The model under review builds one solid part; all positions refer to its coordinate system, in mm. A direction names the side the tool comes from. Coordinates: 2 decimals unless noted, no trailing zeros. Order: outer loops, then holes, each group sorted by start corner. A loop starts at its lowest first (then second) coordinate and runs counter-clockwise, first axis right, second up.
from build123d import *

# Parameters (mm, degrees)
SKETCH_1_W      = 86
SKETCH_1_H      = 57.4
EXTRUDE_1_DEPTH = 1.6
SKETCH_2_W      = 84.66
SKETCH_2_H      = 54.44
EXTRUDE_2_DEPTH = 1.3
SKETCH_3_W      = 75.45
SKETCH_3_H      = 50.61
EXTRUDE_3_DEPTH = 0.1
SKETCH_4_W      = 51.17
SKETCH_4_H      = 5
EXTRUDE_4_DEPTH = 14


with BuildPart() as part:
    # 草图1 → 凸台-拉伸1 (new body)
    with BuildSketch(Plane(origin=(0, 0, 0), x_dir=(1, 0, 0), z_dir=(0, 1, 0))):
        with Locations((-1.791666667, -4.811111111)):
            Rectangle(SKETCH_1_W, SKETCH_1_H)
    extrude(amount=EXTRUDE_1_DEPTH)

    # 草图2 → 凸台-拉伸2 (add)
    with BuildSketch(Plane(origin=(0, 1.6, 0), x_dir=(1, 0, 0), z_dir=(0, 1, 0))):
        with Locations((-1.461666667, -4.611111111)):
            Rectangle(SKETCH_2_W, SKETCH_2_H)
    extrude(amount=EXTRUDE_2_DEPTH)

    # 草图3 → 凸台-拉伸3 (add)
    with BuildSketch(Plane(origin=(0, 2.9, 0), x_dir=(1, 0, 0), z_dir=(0, 1, 0))):
        with Locations((1.323333333, -4.516111111)):
            Rectangle(SKETCH_3_W, SKETCH_3_H)
    extrude(amount=EXTRUDE_3_DEPTH)

    # 草图4 → 凸台-拉伸4 (add)
    with BuildSketch(Plane.XZ):
        with Locations((-11.666666667, -19.698888889)):
            Rectangle(SKETCH_4_W, SKETCH_4_H)
    extrude(amount=EXTRUDE_4_DEPTH)


solid = part.part
(1) Consider section C-C (y = -8.25). Give the boundary of the cut face in (x, z).
(2) Consider section A-A (z = 19.5). Give the boundary of the cut face in (x, y).
(3) Insertion check: pin 1 Ø1 at (x, y) = (-10.5, -3) entering from -Z; pin 2 Ø6 at (x, z) = (-13, -7.5) entering from -Y; pin 3 Ø0.7 at (y, z) = (2.5, 9.5) entering from +X. Each pin has a flat end and moves straight along its axis. Give the tip position at first contact, or say it passes through.
(4) Consider section B-B (x = -30.5). Give the boundary of the cut face in (y, z), then the cut area to 3 significant figures.
(5) Tool access review of faces 1 (the face through (-12, -7, -22.199)), 2 (the face through (-37.252, -7, -20)), 3 (the face through (-11, 2.9, 31)), 4 (the face through (13.918, -7, -20)): name each direction out of +Z, -Z, +X, -X, +Y, -Y from which nothing blocks a thin tool from reaching the whole face with its end or side.
(6) Wall thickness on line 1 (Y direction, x = -7.5, z = -9.5); line 2 (Z direction, x = 0, y = -4); line 3 (Z direction, x = -41, y = 2): over which ranges is each line inside the solid? List them lowest first.
Findings:
1. outline: (-37.25, -22.2) - (13.92, -22.2) - (13.92, -17.2) - (-37.25, -17.2) - close
2. outline: (-44.79, 0) - (41.21, 0) - (41.21, 1.6) - (40.87, 1.6) - (40.87, 2.9) - (39.05, 2.9) - (39.05, 3) - (-36.4, 3) - (-36.4, 2.9) - (-43.79, 2.9) - (-43.79, 1.6) - (-44.79, 1.6) - close
3. pin 1: stops at z = -22.2
3. pin 2: stops at y = 0
3. pin 3: stops at x = 40.87
4. outline: (-14, -22.2) - (0, -22.2) - (0, -23.89) - (1.6, -23.89) - (1.6, -22.61) - (2.9, -22.61) - (2.9, -20.79) - (3, -20.79) - (3, 29.82) - (2.9, 29.82) - (2.9, 31.83) - (1.6, 31.83) - (1.6, 33.51) - (0, 33.51) - (0, -17.2) - (-14, -17.2) - close
4. area: 238 mm2
5. face 1: -Z, +X, -X, -Y
5. face 2: +Z, -Z, -X, -Y
5. face 3: +Y
5. face 4: +Z, -Z, +X, -Y
6. line 1: y = 0 to 3
6. line 2: z = -22.2 to -17.2
6. line 3: z = -22.61 to 31.83
